Here's how the part is built. I have some questions about the finished solid (model axes, mm). Give positions to 0.01 mm unless a question says otherwise; leave off trailing zeros. Loops run counter-clockwise (first coordinate to the right, second up) from the corner with the lowest first, then second, coordinate; pieces in that order, holes last. Notation, with made-up numbers: (77.5, 83) - (103.5, 83) arc R28 ccw to (103.5, 104) - close; hole circle Ø6 at (-36.75, -9.5). An arc over 180 degrees is marked (long way). Use one line per item in the form item = value.
from build123d import *

# Parameters (mm, degrees)
FILLET4_R = 2
FILLET5_R = 2
FILLET6_R = 2
FILLET7_R = 2


# Some blends are built 0.0001 mm under size
with BuildPart() as part:
    # Sketch2 → Revolve1 (revolve)
    with BuildSketch(Plane.XY, mode=Mode.PRIVATE) as revolve1_sk:
        with BuildLine():
            Line((0, 0), (0, 12))
            Line((0, 12), (17, 12))
            Line((17, 12), (17, 11.196152423))
            ThreePointArc((17, 11.196152423), (14, 6), (17, 0.803847577))
            Line((17, 0.803847577), (17, 0))
            Line((17, 0), (0, 0))
        make_face()
    revolve(revolve1_sk.sketch.rotate(Axis((0, 0, 0), (0, 1, 0)), 90), axis=Axis((0, 0, 0), (0, 1, 0)))

    # Fillet4
    # the kernel refuses this fillet: 2 mm, written as the material it takes off along each edge
    with BuildSketch(Plane(origin=(0, 12, 0), x_dir=(0, 0, -1), z_dir=(1, 0, 0))) as fillet4_piece_1:
        with BuildLine():
            CenterArc((15.397121532, -2), FILLET4_R, 36.732240325, 53.267759675)
            Line((17, -0.803847577), (17.032057569, -0.779924529))
            ThreePointArc((17.032057569, -0.779924529), (17.04, -0.401923789), (17.04, 0))
            Line((17.04, 0), (17, 0.04))
            Line((17, 0.04), (15.397121532, 0.04))
            Line((15.397121532, 0.04), (15.397121532, 0))
        make_face()
    revolve(axis=Axis((0, 12, 0), (0, 1, 0)), mode=Mode.SUBTRACT)

    # Fillet5
    fillet5_edges = [part.edges().sort_by_distance(p)[0] for p in [
        (0, 11.196152423, 17),
    ]]
    fillet(fillet5_edges, radius=FILLET5_R - 0.0001)  # a hair under: the kernel refuses the full size

    # Fillet6
    # the kernel refuses this fillet: 2 mm, written as the material it takes off along each edge
    with BuildSketch(Plane(origin=(0, 0, 0), x_dir=(0, 0, -1), z_dir=(1, 0, 0))) as fillet6_piece_1:
        with BuildLine():
            CenterArc((15.397121532, 2), FILLET6_R, 270, 53.267759675)
            Line((15.397121532, 0), (15.397121532, -0.04))
            Line((15.397121532, -0.04), (17, -0.04))
            Line((17, -0.04), (17.04, 0))
            ThreePointArc((17.04, 0), (17.04, 0.401923789), (17.032057569, 0.779924529))
            Line((17.032057569, 0.779924529), (17, 0.803847577))
        make_face()
    revolve(axis=Axis((0, 0, 0), (0, 1, 0)), mode=Mode.SUBTRACT)

    # Fillet7
    fillet7_edges = [part.edges().sort_by_distance(p)[0] for p in [
        (0, 0.803847577, 17),
    ]]
    fillet(fillet7_edges, radius=FILLET7_R)


solid = part.part
(1) If I drill on probe 1 along Z at (x, y) = (5, 6); probe 2 along X at (y, z) = (10.5, -2.5); probe 3 along Z at (x, y) = (10, 3.5), over which ranges is the centre line in solid material (lowest first)?
Geometry says:
probe_1 = -13.08 to 13.08
probe_2 = -14.8 to 14.8
probe_3 = -10.56 to 10.56
(2) If we section it at A-A (y = 6): List the corners of the cut face in (x, z) for me, plus the area to 3 significant figures.
Geometry says:
outline = circle Ø28 at (0, 0)
area = 616 mm²
(3) For P1, Ø1.5, axis at y = 2.5, z = 7.5, coming from the -X side; P2, Ø4, axis at y = 10.5, z = 9, coming from the +X side; P3, Ø4, axis at x = 12, y = 8, coming from the -Z side, each with a flat end and sliding along its axis, tell me the tip position at first contact or that it passes through.
Geometry says:
P1 = -13.44
P2 = 13.33
P3 = -10.68
